For this review, use the dimensioned drawing (mm, ordinates from the lowest corner) and the shaded views. A direction names the side the tool comes from. Round coordinates to 2 decimals unless told otherwise and drop trailing zeros. Order: outer loops, then holes, each group sorted by start corner. A loop starts at its lowest first (then second) coordinate and runs counter-clockwise, first axis right, second up. Notation, with made-up numbers: (1, 62.25) - (33, 62.25) arc R15 ccw to (33, 82.25) - close; hole circle Ø4 at (63.5, 69.5). An arc over 180 degrees is marked (long way). Write item = value, one per line.
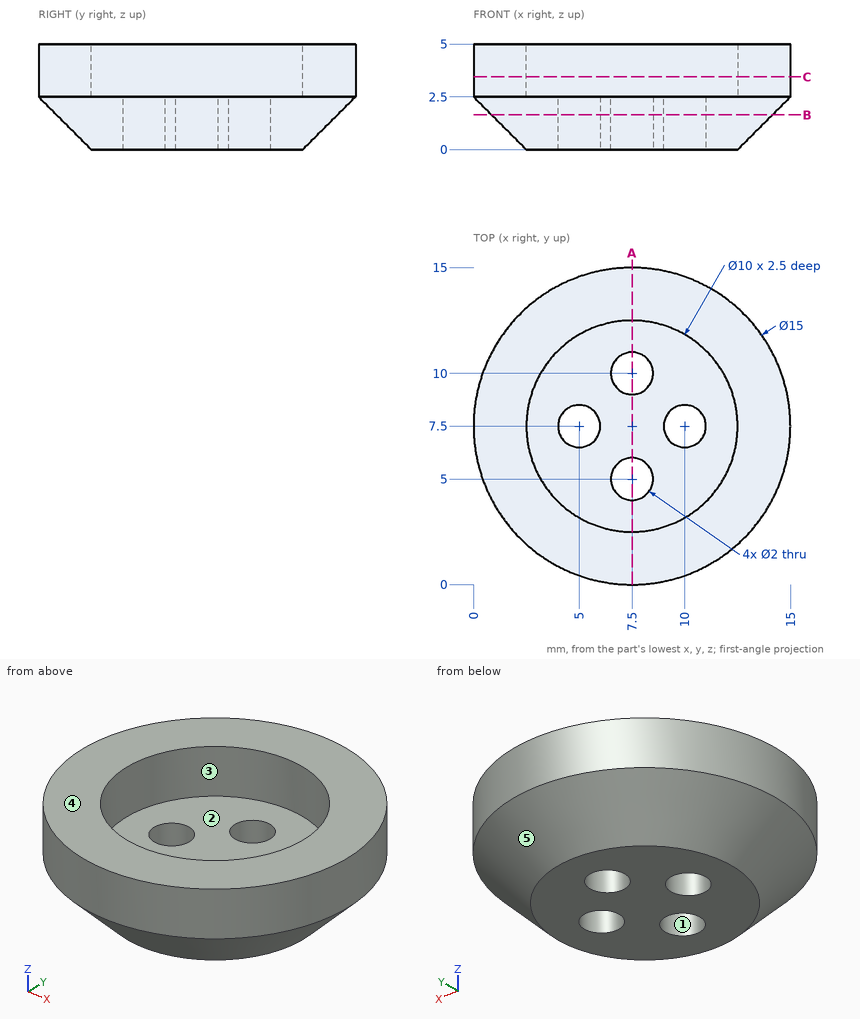
Item 1: Take a section at B-B, the plane z = 1.65. State the section outline as (x, y) points.
Data:
outline = circle Ø13.3 at (7.5, 7.5); hole circle Ø2 at (5, 7.5); hole circle Ø2 at (7.5, 5); hole circle Ø2 at (7.5, 10); hole circle Ø2 at (10, 7.5)
Item 2: Take a section at A-A, the plane x = 7.5. State the section outline as (y, z) points, and give its area (4 significant figures).
Data:
outline = (0, 2.5) - (2.5, 0) - (4, 0) - (4, 2.5) - (2.5, 2.5) - (2.5, 5) - (0, 5) - close; (6, 0) - (9, 0) - (9, 2.5) - (6, 2.5) - close; (11, 0) - (12.5, 0) - (15, 2.5) - (15, 5) - (12.5, 5) - (12.5, 2.5) - (11, 2.5) - close
area = 33.75 mm2
Item 3: Insertion check: P1, Ø3, axis at x = 5, y = 7.5, coming from the +Z side; P2, Ø1.5, axis at y = 13, z = 3, coming from the -X side; P3, Ø2, axis at x = 4.5, z = 4, coming from the +Y side. Each pin has a flat end and moves straight along its axis. Give the tip position at first contact, or say it passes through.
Data:
P1 = 2.5
P2 = 1.7
P3 = 14.73
Item 4: For the marked faces 1 and 2, list the 3-axis set-ups (+Z, -Z, +X, -X, +Y, -Y) from which the entire face can be reached by the end or side of a thin tool; tool diameter is ignored.
Data:
face_1 = +Z, -Z
face_2 = +Z
Item 5: For line 1 along Z through (x, y) = (11.5, 9); line 2 along Y through (x, z) = (10.25, 3.7); line 3 along Y through (x, z) = (7.75, 1.2), list the stretches that pass through material, from the lowest coordinate up. Write a range as [from, to].
Data:
line_1 = [0, 2.5]
line_2 = [0.52, 3.32], [11.68, 14.48]
line_3 = [1.31, 4.03], [5.97, 9.03], [10.97, 13.69]
Item 6: The part is to be moulded in two halves that separate along Y. For the marked faces 3, 4 and 5, say which applies: +Y half, -Y half, draft (parallel to the pull), parting line (faces both ways), or undercut.
Data:
face_3 = undercut
face_4 = draft
face_5 = parting line
Item 7: Take a section at C-C, the plane z = 3.45. State the section outline as (x, y) points.
Data:
outline = circle Ø15 at (7.5, 7.5); hole circle Ø10 at (7.5, 7.5)
